Model file for the job. Use its own axes, mm. Face numbers are marked on the shaded views. A direction names the side the tool comes from. Round coordinates to 2 decimals unless told otherwise and drop trailing zeros. Order: outer loops, then holes, each group sorted by start corner. A loop starts at its lowest first (then second) coordinate and runs counter-clockwise, first axis right, second up. Notation, with made-up numbers: (-16.75, 25) -> (-3.75, 25) arc R33 cw to (-3.75, 61) -> close; hole circle Ø3 at (75.25, 31). An arc over 180 degrees is marked (long way). Put each result on its own line as item: value. Start each with the question number.
Q1. 3-axis set-ups, long thin cutter, end or side, ignore diameter. For the marked faces 4 and 5: which of +Z, -Z, +X, -X, +Y, -Y reach the whole face in a straight line?
Q2. Cut at B-B, the plane y = 155. State how many separate pieces and enclosed holes the cut face has, and give its area (3 significant figures).
Q3. Cut at A-A, the plane x = 402. List the corners of the cut face in (y, z).
Q4. Flat gauge pins, fed straight in: P1, Ø3, axis at x = 300, y = 148, coming from the -Z side; P2, Ø3, axis at x = 323, y = 149, coming from the +Z side; P3, Ø3, axis at x = 296.5, z = -7, coming from the +Y side; P4, Ø9.5, axis at x = 208.88, y = 155, coming from the +Z side. Where does each tip first touch, or does it go through?
Q5. Cut at D-D, the plane z = -0.75. List the corners of the cut face in (x, y), and give its area (3 significant figures).
Q6. Pull direction Z, two halves, no side cores. Call the marked faces 1, 2 and 3: released by +Z, released by -Z, zero draft, split by the parting line, or undercut.
Q7. Cut at C-C, the plane x = 352.5. List the corners of the cut face in (y, z), and give its area (3 significant figures).
Q8. Probe L1, parallel to X at y = 155, z = 8.15; L2, parallel to Z at x = 381.5, y = 152.75; L3, parallel to X at y = 151.5, z = 7.75. List the from-to ranges inside material, lowest first.
from build123d import *

# Parameters (mm, degrees)
ESBO_O1_R                = 4.15
RESSALTO_EXTRUS_O1_DEPTH = 10
ESBO_O2_W                = 41
ESBO_O2_H                = 11
CORTE_EXTRUS_O1_DEPTH    = 421.865295251
FILETE1_R                = 2
ESBO_O3_W                = 41
ESBO_O3_H                = 11
CORTE_EXTRUS_O2_DEPTH    = 421.865295251
ESBO_O4_W                = 130
ESBO_O4_H                = 51.333908156
CORTE_EXTRUS_O3_DEPTH    = 452.376336051
RESSALTO_EXTRUS_O2_DEPTH = 130
FILETE2_R                = 9
FILETE3_R                = 2


with BuildPart() as part:
    # Esbo_o1 → Ressalto-extrus_o1 (new, symmetric)
    with BuildSketch(Plane.XY):
        with BuildLine():
            Line((208.88140452, 163), (412.442144352, 163))
            ThreePointArc((412.442144352, 163), (420.442144352, 155), (412.442144352, 147))
            Line((412.442144352, 147), (208.88140452, 147))
            ThreePointArc((208.88140452, 147), (200.88140452, 155), (208.88140452, 163))
        make_face()
        with Locations((208.88140452, 155)):
            Circle(ESBO_O1_R, mode=Mode.SUBTRACT)
        with Locations((412.442144352, 155)):
            Circle(ESBO_O1_R, mode=Mode.SUBTRACT)
    extrude(amount=RESSALTO_EXTRUS_O1_DEPTH, both=True)

    # Esbo_o2 → Corte-extrus_o1 (cut, through all)
    with BuildSketch(Plane(origin=(0, 163, 0), x_dir=(1, 0, 0), z_dir=(0, 1, 0))):
        with Locations((221.38140452, 0)):
            Rectangle(ESBO_O2_W, ESBO_O2_H)
    extrude(amount=-CORTE_EXTRUS_O1_DEPTH, mode=Mode.SUBTRACT)

    # Filete1
    filete1_edges = [part.edges().sort_by_distance(p)[0] for p in [
        (241.88140452, 155, 5.5),
        (241.88140452, 155, -5.5),
    ]]
    fillet(filete1_edges, radius=FILETE1_R)

    # Esbo_o3 → Corte-extrus_o2 (cut, through all)
    with BuildSketch(Plane(origin=(0, 163, 0), x_dir=(1, 0, 0), z_dir=(0, 1, 0))):
        with Locations((399.942144352, 0)):
            Rectangle(ESBO_O3_W, ESBO_O3_H)
    extrude(amount=-CORTE_EXTRUS_O2_DEPTH, mode=Mode.SUBTRACT)

    # Esbo_o4 → Corte-extrus_o3 (cut, through all)
    with BuildSketch(Plane.XY.offset(10)):
        with Locations((310.661774436, 149.883332027)):
            Rectangle(ESBO_O4_W, ESBO_O4_H)
    extrude(amount=-CORTE_EXTRUS_O3_DEPTH, mode=Mode.SUBTRACT)


with BuildPart() as corte_extrus_o3_piece_1:
    # of the separate pieces the step leaves, piece 1, a body of its own (corte_extrus_o3_pieces)
    add(part.part.solids().sort_by_distance((241.88140452, 163, -3.5))[0])



with BuildPart() as corte_extrus_o3_piece_2:
    # of the separate pieces the step leaves, piece 2, a body of its own (corte_extrus_o3_pieces)
    add(part.part.solids().sort_by_distance((375.661774436, 163, -10))[0])


with BuildPart() as corte_extrus_o3_piece_1_1:
    add(corte_extrus_o3_piece_1.part)

    add(corte_extrus_o3_piece_2.part)  # Ressalto-extrus_o2 merges Corte-extrus_o3 piece 2
    # Esbo_o5 → Ressalto-extrus_o2 (add)
    with BuildSketch(Plane(origin=(245.661774436, 0, 0), x_dir=(0, 0, -1), z_dir=(1, 0, 0))):
        Polygon((-4, 147), (-4, 151), (-10, 151), (-10, 159), (-4, 159), (-4, 163), (4, 163), (4, 159), (10, 159), (10, 151), (4, 151), (4, 147), align=None)
    extrude(amount=RESSALTO_EXTRUS_O2_DEPTH)

    # Filete2
    # the kernel refuses this fillet: 9 mm, written as the material it adds along each edge
    with BuildSketch(Plane(origin=(375.661774436, 151, -10), x_dir=(0, -1, 0), z_dir=(0, 0, 1))) as filete2_piece_1_section:
        with BuildLine():
            CenterArc((9, -7.483314774), FILETE2_R, 123.748988596, 56.251011404)
            Line((0, -7.483314774), (-0.18, -7.483314774))
            Line((-0.18, -7.483314774), (-0.18, 0))
            Line((-0.18, 0), (0, 0.18))
            ThreePointArc((0, 0.18), (2, 0.18), (3.9, 0.149666295))
            Line((3.9, 0.149666295), (4, 0))
        make_face()
    filete2_piece_1 = extrude(amount=24.708286934, mode=Mode.PRIVATE)
    filete2_piece_1 = split(filete2_piece_1, bisect_by=Plane(origin=(373.762740139, 149.968595049, 10), z_dir=(0, 0, -1)), keep=Keep.TOP, mode=Mode.PRIVATE)
    add(filete2_piece_1)
    with BuildSketch(Plane(origin=(375.661774436, 151, -14.708286934), x_dir=(0, -1, 0), z_dir=(0, 0, 1))) as filete2_piece_2_section:
        with BuildLine():
            CenterArc((9, -7.483314774), FILETE2_R, 123.748988596, 56.251011404)
            Line((0, -7.483314774), (-0.18, -7.483314774))
            Line((-0.18, -7.483314774), (-0.18, 0))
            Line((-0.18, 0), (0, 0.18))
            ThreePointArc((0, 0.18), (2, 0.18), (3.9, 0.149666295))
            Line((3.9, 0.149666295), (4, 0))
        make_face()
    filete2_piece_2 = extrude(amount=24.708286934, mode=Mode.PRIVATE)
    filete2_piece_2 = split(filete2_piece_2, bisect_by=Plane(origin=(373.762740139, 149.968595049, -10), z_dir=(0, 0, 1)), keep=Keep.TOP, mode=Mode.PRIVATE)
    add(filete2_piece_2)
    with BuildSketch(Plane(origin=(375.661774436, 159, 10), x_dir=(0, 1, 0), z_dir=(0, 0, -1))) as filete2_piece_3_section:
        with BuildLine():
            CenterArc((9, -7.483314774), FILETE2_R, 123.748988596, 56.251011404)
            Line((0, -7.483314774), (-0.18, -7.483314774))
            Line((-0.18, -7.483314774), (-0.18, 0))
            Line((-0.18, 0), (0, 0.18))
            ThreePointArc((0, 0.18), (2, 0.18), (3.9, 0.149666295))
            Line((3.9, 0.149666295), (4, 0))
        make_face()
    filete2_piece_3 = extrude(amount=24.708286934, mode=Mode.PRIVATE)
    filete2_piece_3 = split(filete2_piece_3, bisect_by=Plane(origin=(373.762740139, 160.031404951, -10), z_dir=(0, 0, 1)), keep=Keep.TOP, mode=Mode.PRIVATE)
    add(filete2_piece_3)
    with BuildSketch(Plane(origin=(375.661774436, 159, 14.708286934), x_dir=(0, 1, 0), z_dir=(0, 0, -1))) as filete2_piece_4_section:
        with BuildLine():
            CenterArc((9, -7.483314774), FILETE2_R, 123.748988596, 56.251011404)
            Line((0, -7.483314774), (-0.18, -7.483314774))
            Line((-0.18, -7.483314774), (-0.18, 0))
            Line((-0.18, 0), (0, 0.18))
            ThreePointArc((0, 0.18), (2, 0.18), (3.9, 0.149666295))
            Line((3.9, 0.149666295), (4, 0))
        make_face()
    filete2_piece_4 = extrude(amount=24.708286934, mode=Mode.PRIVATE)
    filete2_piece_4 = split(filete2_piece_4, bisect_by=Plane(origin=(373.762740139, 160.031404951, 10), z_dir=(0, 0, -1)), keep=Keep.TOP, mode=Mode.PRIVATE)
    add(filete2_piece_4)
    with BuildSketch(Plane(origin=(245.661774436, 151, -10), x_dir=(1, 0, 0), z_dir=(0, 0, 1))) as filete2_piece_5_section:
        with BuildLine():
            CenterArc((7.483314774, -9), FILETE2_R, 90, 56.251011404)
            Line((0, -4), (-0.149666295, -3.9))
            ThreePointArc((-0.149666295, -3.9), (-0.18, -2), (-0.18, 0))
            Line((-0.18, 0), (0, 0.18))
            Line((0, 0.18), (7.483314774, 0.18))
            Line((7.483314774, 0.18), (7.483314774, 0))
        make_face()
    filete2_piece_5 = extrude(amount=24.708286934, mode=Mode.PRIVATE)
    filete2_piece_5 = split(filete2_piece_5, bisect_by=Plane(origin=(247.560808733, 149.968595049, 10), z_dir=(0, 0, -1)), keep=Keep.TOP, mode=Mode.PRIVATE)
    add(filete2_piece_5)
    with BuildSketch(Plane(origin=(245.661774436, 151, -14.708286934), x_dir=(1, 0, 0), z_dir=(0, 0, 1))) as filete2_piece_6_section:
        with BuildLine():
            CenterArc((7.483314774, -9), FILETE2_R, 90, 56.251011404)
            Line((0, -4), (-0.149666295, -3.9))
            ThreePointArc((-0.149666295, -3.9), (-0.18, -2), (-0.18, 0))
            Line((-0.18, 0), (0, 0.18))
            Line((0, 0.18), (7.483314774, 0.18))
            Line((7.483314774, 0.18), (7.483314774, 0))
        make_face()
    filete2_piece_6 = extrude(amount=24.708286934, mode=Mode.PRIVATE)
    filete2_piece_6 = split(filete2_piece_6, bisect_by=Plane(origin=(247.560808733, 149.968595049, -10), z_dir=(0, 0, 1)), keep=Keep.TOP, mode=Mode.PRIVATE)
    add(filete2_piece_6)
    with BuildSketch(Plane(origin=(245.661774436, 159, 14.708286934), x_dir=(1, 0, 0), z_dir=(0, 0, -1))) as filete2_piece_7_section:
        with BuildLine():
            CenterArc((7.483314774, -9), FILETE2_R, 90, 56.251011404)
            Line((0, -4), (-0.149666295, -3.9))
            ThreePointArc((-0.149666295, -3.9), (-0.18, -2), (-0.18, 0))
            Line((-0.18, 0), (0, 0.18))
            Line((0, 0.18), (7.483314774, 0.18))
            Line((7.483314774, 0.18), (7.483314774, 0))
        make_face()
    filete2_piece_7 = extrude(amount=24.708286934, mode=Mode.PRIVATE)
    filete2_piece_7 = split(filete2_piece_7, bisect_by=Plane(origin=(247.560808733, 160.031404951, 10), z_dir=(0, 0, -1)), keep=Keep.TOP, mode=Mode.PRIVATE)
    add(filete2_piece_7)
    with BuildSketch(Plane(origin=(245.661774436, 159, 10), x_dir=(0, 1, 0), z_dir=(0, 0, -1))) as filete2_piece_8_section:
        with BuildLine():
            CenterArc((9, 7.483314774), FILETE2_R, 180, 56.251011404)
            Line((0, 7.483314774), (-0.18, 7.483314774))
            Line((-0.18, 7.483314774), (-0.18, 0))
            Line((-0.18, 0), (0, -0.18))
            ThreePointArc((0, -0.18), (2, -0.18), (3.9, -0.149666295))
            Line((3.9, -0.149666295), (4, 0))
        make_face()
    filete2_piece_8 = extrude(amount=24.708286934, mode=Mode.PRIVATE)
    filete2_piece_8 = split(filete2_piece_8, bisect_by=Plane(origin=(247.560808733, 160.031404951, -10), z_dir=(0, 0, 1)), keep=Keep.TOP, mode=Mode.PRIVATE)
    add(filete2_piece_8)

    # Filete3
    filete3_edges = [corte_extrus_o3_piece_1_1.edges().sort_by_distance(p)[0] for p in [
        (379.442144352, 155, 5.5),
        (379.442144352, 155, -5.5),
    ]]
    fillet(filete3_edges, radius=FILETE3_R)


solid = corte_extrus_o3_piece_1_1.part
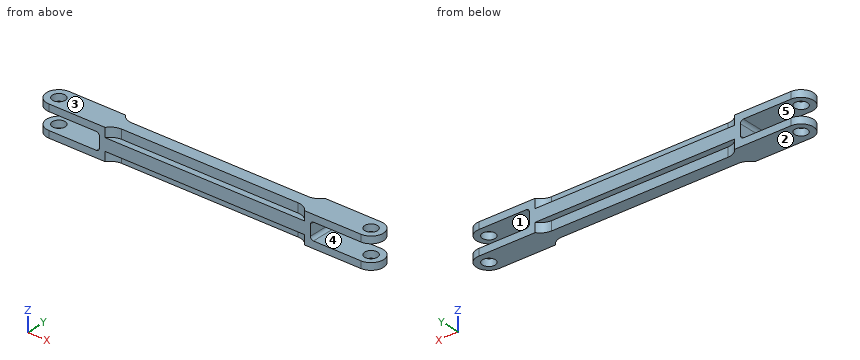
Ans:
1. face 4: +X, +Y, -Y
1. face 5: -X, +Y, -Y
2. separate pieces: 5
2. enclosed holes: 0
2. area: 3,340 mm^2
3. outline: (147, -10) -> (163, -10) -> (163, -5.5) -> (147, -5.5) -> close; (147, 5.5) -> (163, 5.5) -> (163, 10) -> (147, 10) -> close
4. P1: stops at z = -4
4. P2: stops at z = 4
4. P3: stops at y = 159
4. P4: stops at z = 10
5. outline: (241.88, 147) -> (379.44, 147) -> (379.44, 163) -> (241.88, 163) -> close
5. area: 2,200 mm^2
6. face 1: undercut
6. face 2: released by -Z
6. face 3: released by +Z
7. outline: (147, -4) -> (151, -4) -> (151, -10) -> (159, -10) -> (159, -4) -> (163, -4) -> (163, 4) -> (159, 4) -> (159, 10) -> (151, 10) -> (151, 4) -> (147, 4) -> close
7. area: 224 mm^2
8. L1: x = 200.88 to 204.73, 213.03 to 408.29, 416.59 to 420.44
8. L2: z = -10 to -5.5, 5.5 to 10
8. L3: x = 201.69 to 206.65, 211.11 to 410.21, 414.67 to 419.64
